Geometry: final body of the model. Coordinates: model frame, mm. A direction names the side the tool comes from. Give positions to 0.01 mm unless a question says otherwise; leave off trailing zeros. Write each loop counter-clockwise with the first axis right and the second up, starting at its lowest first coordinate (ties: lowest second). Pieces come first, ordered by that corner, then holes.
Q1. Cut plane A-A on x = 69. Return the cut outline in (y, z) (3 decimals).
Q2. Reachability of faces 1 (the face through (3, -2.6, 8)), 2 (the face through (35, -3, 7.5)), 3 (the face through (35, -5.81, 3)) from +Z, -Z, +X, -X, +Y, -Y: full face, straight path, thin tool, end or side. Return the list, or none.
Q3. Pin query (flat end, axial travel): pin 1 (0.7 mm diameter, centred on y = -5.5, z = 15.5, fed in from -X); pin 2 (1.6 mm diameter, centred on y = -3.5, z = 2.5, fed in from +X); pin 3 (1.5 mm diameter, centred on x = 56, z = 9, fed in from +Y); pin 4 (4 mm diameter, centred on x = 11, z = 7.5, fed in from -Y). Return the tip coordinate at first contact, or that it passes through.
Q4. Line query: L1, parallel to Z at x = 2.5, y = -1.3 (3 decimals); L2, parallel to Z at x = 14, y = -0.5; L3, parallel to Y at x = 20.5, z = 1.25. Output: solid intervals per line, ascending.
Q5. Draft query along X for faces 4 (the face through (66.25, -4, 4)), 5 (the face through (35.323, -5.084, 15.117)), 6 (the face through (5, -1, 11)), 7 (the face through (70.25, -1.41, 4.39)). Return one class per face: pulls with the +X half, pulls with the -X half, needs draft (parallel to the pull), parting line crosses it, or undercut.
Q6. Cut plane B-B on z = 10. Return the cut outline in (x, y), plus the area to 3 significant figures.
Q7. Cut plane D-D on x = 47.5. Return the cut outline in (y, z).
Q8. Cut plane C-C on y = -2. Return the cut outline in (x, z) (3 decimals).
```python
from build123d import *

# Parameters (mm, degrees)
BOSS_EXTRUDE1_DEPTH = 71.5
SKETCH2_R           = 1.35
CUT_EXTRUDE1_DEPTH  = 6.81
BOSS_EXTRUDE2_DEPTH = 2.6
BOSS_EXTRUDE3_DEPTH = 61
SKETCH5_W           = 5.25
SKETCH5_H           = 3.21
CUT_EXTRUDE2_DEPTH  = 17.5
FILLET1_R           = 1
CHAMFER1_SIZE       = 0.25


with BuildPart() as part:
    # Sketch1 → Boss-Extrude1 (new body)
    with BuildSketch(Plane(origin=(0, 0, 0), x_dir=(0, 0, -1), z_dir=(1, 0, 0))):
        Polygon((0, 0), (-7.5, 0), (-7.5, -5.15), (-6.25, -5.15), (-6.25, -5.81), (0, -5.81), align=None)
    extrude(amount=BOSS_EXTRUDE1_DEPTH)

    # Sketch2 → Cut-Extrude1 (cut, through all)
    with BuildSketch(Plane(origin=(0, 0, 0), x_dir=(1, 0, 0), z_dir=(0, 1, 0))):
        with Locations((2.5, -3.875)):
            Circle(SKETCH2_R)
        with Locations((69, -3.875)):
            Circle(SKETCH2_R)
    extrude(amount=-CUT_EXTRUDE1_DEPTH, mode=Mode.SUBTRACT)

    # Sketch3 → Boss-Extrude2 (add)
    with BuildSketch(Plane(origin=(0, 0, 0), x_dir=(1, 0, 0), z_dir=(0, 1, 0))):
        Polygon((0, -7.5), (0, -16.5), (71.5, -16.5), (71.5, -7.5), (66.5, -7.5), (66.5, -14.23), (5, -14.23), (5, -7.5), align=None)
    extrude(amount=-BOSS_EXTRUDE2_DEPTH)

    # Sketch4 → Boss-Extrude3 (add)
    with BuildSketch(Plane.ZY.offset(-5.25)):
        Polygon((16.5, -2.6), (16.5, -7.5), (15.98, -7.5), (14.23, -2.6), align=None)
    extrude(amount=-BOSS_EXTRUDE3_DEPTH)

    # Sketch5 → Cut-Extrude2 (cut, through all)
    with BuildSketch(Plane(origin=(0, 0, 0), x_dir=(-1, 0, 0), z_dir=(0, 0, -1))):
        with Locations((-2.625, -4.205)):
            Rectangle(SKETCH5_W, SKETCH5_H)
        with Locations((-68.875, -4.205)):
            Rectangle(SKETCH5_W, SKETCH5_H)
    extrude(amount=-CUT_EXTRUDE2_DEPTH, mode=Mode.SUBTRACT)

    # Fillet1
    fillet1_edges = [part.edges().sort_by_distance(p)[0] for p in [
        (71.5, -1.3, 16.5),
        (0, -1.3, 16.5),
        (0, -1.3, 0),
        (71.5, -1.3, 0),
    ]]
    fillet(fillet1_edges, radius=FILLET1_R)

    # Chamfer1
    chamfer1_edges = [part.edges().sort_by_distance(p)[0] for p in [
        (1.15, 0, 3.875),
        (67.65, 0, 3.875),
    ]]
    chamfer(chamfer1_edges, length=CHAMFER1_SIZE)


solid = part.part
```
Data:
1. outline: (-2.6, 0) - (0, 0) - (0, 2.275) - (-0.25, 2.525) - (-2.6, 2.525) - close; (-2.6, 5.225) - (-0.25, 5.225) - (0, 5.475) - (0, 16.5) - (-2.6, 16.5) - close
2. face 1: +Z, -Z, -X, -Y
2. face 2: +Y, -Y
2. face 3: -Z, +X, -X, -Y
3. pin 1: stops at x = 5.25
3. pin 2: stops at x = 66.25
3. pin 3: passes through
3. pin 4: stops at y = -5.81
4. L1: z = 0 to 2.525, 5.225 to 16.5
4. L2: z = 0 to 7.5, 14.23 to 16.5
4. L3: y = -5.81 to 0
5. face 4: pulls with the +X half
5. face 5: needs draft
5. face 6: undercut
5. face 7: undercut
6. outline: (0, -2.6) - (5, -2.6) - (5, 0) - (0, 0) - close; (66.5, -2.6) - (71.5, -2.6) - (71.5, 0) - (66.5, 0) - close
6. area: 26.0 mm2
7. outline: (-7.5, 15.98) - (-2.6, 14.23) - (0, 14.23) - (0, 16.5) - (-7.5, 16.5) - close; (-5.81, 0) - (0, 0) - (0, 7.5) - (-5.15, 7.5) - (-5.15, 6.25) - (-5.81, 6.25) - close
8. outline: (0, 1) arc R1 ccw to (1, 0) - (70.5, 0) arc R1 ccw to (71.5, 1) - (71.5, 15.5) arc R1 ccw to (70.5, 16.5) - (1, 16.5) arc R1 ccw to (0, 15.5) - close; hole circle Ø2.7 at (2.5, 3.875); hole (5, 7.5) - (66.5, 7.5) - (66.5, 14.23) - (5, 14.23) - close; hole circle Ø2.7 at (69, 3.875)
